Autodesk Inventor part; units mm, degrees
ref_plane "YZ Plane" through (0, 0, 0) normal (1, 0, 0) x (0, 1, 0)
ref_plane "XZ Plane" through (0, 0, 0) normal (0, 1, 0) x (-1, 0, 0)
ref_plane "XY Plane" through (0, 0, 0) normal (0, 0, 1) x (1, 0, 0)
sketch "Sketch1" plane through (0, 0, 0) normal (0, 0, 1) x (1, 0, 0)
  line L0 (-18, 0) -> (18, 0) construction
  arc A0 (-18, 3.8571) -> (-18, -3.8571) centre (-18, 0) ccw
  arc A1 (18, -3.8571) -> (18, 3.8571) centre (18, 0) ccw
  line L1 (-18, -3.8571) -> (18, -3.8571)
  line L2 (18, 3.8571) -> (-18, 3.8571)
  point P0 (0, 0)
  dimension "d26" = 36
extrude "Extrusion1" add sketch "Sketch1" along normal blind 7
sketch "Sketch2" plane through (-18, 3.8571, 0) normal (0, 1, 0) x (1, 0, 0)
  line L0 (33, -4) -> (50.7344, -4) construction
  line L1 (36, -7) -> (0, -7)
  line L2 (10, -3) -> (26, -3)
  line L3 (28, -5) -> (28, -7)
  line L4 (28, -7) -> (8, -7)
  line L5 (8, -7) -> (8, -5)
  line L6 (36, 0) -> (0, 0)
  line L7 (0, 0) -> (0, -7)
  line L8 (36, 0) -> (36, -7)
  line L9 (3, -4) -> (-4.7246, -4)
  line L10 (-4.7246, -4) -> (-4.7246, 3)
  line L11 (-4.7246, 3) -> (5, 3)
  line L12 (5, 3) -> (5, -2)
  line L13 (33, -4) -> (47.7116, -4)
  line L14 (47.7116, -4) -> (47.7116, 0.5212)
  line L15 (47.7116, 0.5212) -> (31, 0.5212)
  line L16 (31, 0.5212) -> (31, -2)
  arc A0 (3, -4) -> (5, -2) centre (3, -2) ccw
  arc A1 (10, -3) -> (8, -5) centre (10, -5) ccw
  arc A2 (28, -5) -> (26, -3) centre (26, -5) ccw
  arc A3 (31, -2) -> (33, -4) centre (33, -2) ccw
  point P0 (18, 0)
  point P1 (8, -3)
  point P2 (28, -3)
  point P3 (5, -4)
  dimension "d7" = 3
  dimension "d8" = 8
  dimension "d9" = 8
  dimension "d10" = 3
  dimension "d11" = 3
  dimension "d24" = 2
extrude "Extrusion2" cut sketch "Sketch2" against normal blind 10 contours L1 L5 A1 L2 A2 L3 | L13 A3 L16 L6 L8 | L8 L6 L16 L15 L14 L13 | L9 L10 L11 L12 L6 L7 | L7 L6 L12 A0 L9
sketch "Sketch3" plane through (0, 0, 7) normal (0, 0, 1) x (1, 0, 0)
  arc A0 (-18, 3.8571) -> (-18, -3.8571) centre (-18, 0) ccw
  point P0 (0, 0)
sketch "Sketch4" plane through (-13, 3.8571, 4) normal (0, 0, -1) x (-1, 0, 0)
  arc A0 (5, -7.7143) -> (5, 0) centre (5, -3.8571) ccw
  point P0 (-13, -3.8571)
hole "Hole1" at (-18, 0, 4) direction (0, 0, 1) diameter 4 depth 3 tip angle 118 counterbore diameter 5 counterbore depth 0.85
pattern_linear "Rectangular Pattern1" count 2 spacing 36 along (1, 0, 0) of "Hole1"
fillet "Fillet1" radius 2 2 edges at (13, 0, 0) (-13, 0, 0)
properties part number "opencm_strap"
Check sheet for the modelled part. Datum: model origin and axes. Units: mm. A direction names the side the tool comes from. Give positions to 0.01 mm unless a question says otherwise; leave off trailing zeros. Write each loop counter-clockwise with the first axis right and the second up, starting at its lowest first coordinate (ties: lowest second). Pieces come first, ordered by that corner, then holes. Notation, with made-up numbers: (6, 51) - (31, 51) arc R32 ccw to (31, 88) - close; hole circle Ø10 at (-34.5, -6.5). An arc over 180 degrees is marked (long way). Answer as a JSON object with one key per item and string values. Group by question number.
1) Sectioned sample at A-A (z = 5.5). Record the cut outline in (x, y).
2) Sectioned sample at D-D (x = 1). Record the cut outline in (y, z), then the cut area to 3 significant figures.
3) Thickness scan on probe 1 along X at (y, z) = (0, 5.5); probe 2 along Y at (x, z) = (-18, 4.4); probe 3 along X at (y, z) = (0, 4.4). Record the ranges inside material, lowest first. Write a range as from..to.
4) Release check for a two-part mould opening along X. For faces 4 (the face through (-20.48, -0.33, 4.43)), 5 (the face through (20, -2, 4)), 6 (the face through (12.4, -0.05, 0.57)) record: pulls with the +X half, pulls with the -X half, needs draft (parallel to the pull), parting line crosses it, or undercut.
5) Sectioned sample at B-B (y = 0). Give the number of separate pieces and of enclosed holes in the cut face, then the cut area to 3 significant figures.
6) Sectioned sample at C-C (x = -17). Record the cut outline in (y, z).
7) Access from +Z, -Z, +X, -X, +Y, -Y to the whole of each face (thin tool, end or side, straight path). Record for faces 1 (the face through (-20, -1, 4.85)), 2 (the face through (-10, 0, 6)), 3 (the face through (0, 0, 0)).
8) Depth check by flat-ended pin: P1, Ø0.6, axis at y = -1.5, z = 6, coming from the +X side; P2, Ø4, axis at y = 2, z = 2.5, coming from the -X side; P3, Ø2.5, axis at x = 18, y = 1, coming from the -Z side. Enter the tip coordinate at first touch or a pass-through.
Geometry results:
{
 "1": {"outline": "(-18, -3.86) - (-10, -3.86) - (-10, 3.86) - (-18, 3.86) arc R3.86 ccw to start; (10, -3.86) - (18, -3.86) arc R3.86 ccw to (18, 3.86) - (10, 3.86) - close; hole circle Ø4 at (-18, 0); hole circle Ø4 at (18, 0)"},
 "2": {"outline": "(-3.86, 0) - (3.86, 0) - (3.86, 3) - (-3.86, 3) - close", "area": "23.1 mm^2"},
 "3": {"probe 1": "x = -21.86..-20, -16..-10, 10..16, 20..21.86", "probe 2": "y = -3.86..-2.5, 2.5..3.86", "probe 3": "x = -21.86..-20.5, -15.5..-9.91, 9.91..15.5, 20.5..21.86"},
 "4": {"face 4": "undercut", "face 5": "needs draft", "face 6": "pulls with the +X half"},
 "5": {"separate pieces": "3", "enclosed holes": "0", "area": "131 mm^2"},
 "6": {"outline": "(-3.86, 4) - (-2.29, 4) - (-2.29, 4.85) - (-1.73, 4.85) - (-1.73, 7) - (-3.86, 7) - close; (1.73, 4.85) - (2.29, 4.85) - (2.29, 4) - (3.86, 4) - (3.86, 7) - (1.73, 7) - close"},
 "7": {"face 1": "-Z", "face 2": "+Z, +Y, -Y", "face 3": "-Z, +X, -X, +Y, -Y"},
 "8": {"P1": "stops at x = 21.67", "P2": "stops at x = -21.8", "P3": "stops at z = 4.85"}
}
